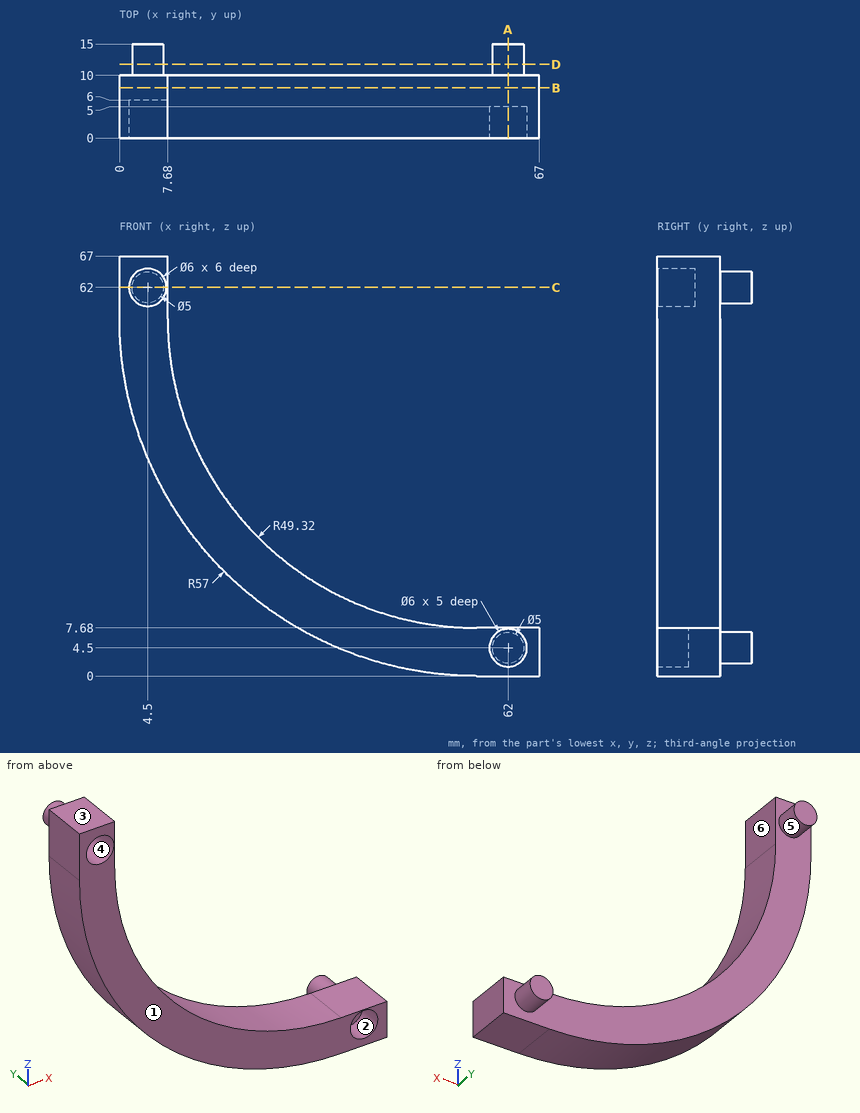
Could you check a few things on this drawing? It's one solid part, dimensions in mm from its lowest x, y, z. A direction names the side the tool comes from. Round coordinates to 2 decimals unless told otherwise and drop trailing zeros. Write each loop counter-clockwise with the first axis right and the second up, starting at its lowest first coordinate (ties: lowest second). Pieces come first, ordered by that corner, then holes. Notation, with made-up numbers: M 78.5,80 L 126.5,80 A13 ccw 126.5,97 Z; hole C 22.25,86 d1. An arc over 180 degrees is marked long. Answer as CSV lines item,"result". Start each with the question number.
1. Suppose I cut it at B-B on y = 8. Write out the boundary of the cut face in (x, z).
2. I need wall thicknesses on probe 1 along X at (y, z) = (3.45, 62); probe 2 along Y at (x, z) = (21.5, 17); probe 3 along X at (y, z) = (1.45, 4.5). Which ranges of each line are inside material? Lowest first, please.
3. I'm going to push flat-ended pins straight in: pin 1 Ø8 at (y, z) = (4.5, 62) entering from +X; pin 2 Ø6 at (y, z) = (12, 30) entering from -X; pin 3 Ø1.5 at (y, z) = (5.5, 16.5) entering from +X. Where does each tip first touch, or does it pass through?
4. Suppose I cut it at D-D on y = 11.75. Write out the boundary of the cut face in (x, z), then the cut area to 3 significant figures.
5. Suppose I cut it at C-C on z = 62. Write out the boundary of the cut face in (x, y).
6. Thinking about a two-plate mould opening in Z: for the marked faces 1, 2 and 3, which applies, released by +Z, released by -Z, zero draft, split by the parting line, or undercut?
7. On a 3-axis mill with a long thin cutter (end or side, diameter ignored), from which of +Z, -Z, +X, -X, +Y, -Y can I reach the whole of each face in a straight line? I mean the marked faces 4, 5 and 6. Say none if no direction works.
8. Suppose I cut it at A-A on x = 62. Write out the boundary of the cut face in (y, z), then the cut area to 3 significant figures.
Check result:
1,outline,"M 0,57 A57 ccw 57,0 L 67,0 L 67,7.68 L 57,7.68 A49.32 cw 7.68,57 L 7.68,67 L 0,67 Z"
2,probe 1,"x = 0 to 1.5, 7.5 to 7.68"
2,probe 2,"y = 0 to 10"
2,probe 3,"x = 34.8 to 59, 65 to 67"
3,pin 1,"stops at x = 7.68"
3,pin 2,"stops at x = 5.66"
3,pin 3,"stops at x = 29.96"
4,outline,"C 4.5,62 d5; C 62,4.5 d5"
4,area,"39.3 mm2"
5,outline,"M 0,0 L 1.5,0 L 1.5,6 L 7.5,6 L 7.5,0 L 7.68,0 L 7.68,10 L 7,10 L 7,15 L 2,15 L 2,10 L 0,10 Z"
6,face 1,"zero draft"
6,face 2,"undercut"
6,face 3,"released by +Z"
7,face 4,"-Y"
7,face 5,"+Y"
7,face 6,"+Z, +X, +Y, -Y"
8,outline,"M 0,0 L 10,0 L 10,2 L 15,2 L 15,7 L 10,7 L 10,7.68 L 0,7.68 L 0,7.5 L 5,7.5 L 5,1.5 L 0,1.5 Z"
8,area,"71.8 mm2"
